```python
from build123d import *

# Parameters (mm, degrees)
SKETCH1_W           = 50
SKETCH1_H           = 10
SKETCH1_R           = 2.25
BOSS_EXTRUDE1_DEPTH = 5
SKETCH3_R           = 2.3
BOSS_EXTRUDE2_DEPTH = 10


with BuildPart() as part:
    # Sketch1 → Boss-Extrude1 (new body)
    with BuildSketch(Plane(origin=(0, 0, 0), x_dir=(1, 0, 0), z_dir=(0, 1, 0))):
        Rectangle(SKETCH1_W, SKETCH1_H)
        with Locations((-20, 0)):
            Circle(SKETCH1_R, mode=Mode.SUBTRACT)
        with Locations((20, 0)):
            Circle(SKETCH1_R, mode=Mode.SUBTRACT)
    extrude(amount=BOSS_EXTRUDE1_DEPTH)

    # Sketch3 → Boss-Extrude2 (add)
    with BuildSketch(Plane.XY.offset(5)):
        with BuildLine():
            Line((-5, 5), (-5, 9))
            ThreePointArc((-5, 9), (0, 14), (5, 9))
            Line((5, 9), (5, 5))
            Line((5, 5), (-5, 5))
        make_face()
        with Locations((0, 9)):
            Circle(SKETCH3_R, mode=Mode.SUBTRACT)
    extrude(amount=-BOSS_EXTRUDE2_DEPTH)


solid = part.part
```
CAD build for the part. Positions are in the model's coordinates, mm. A direction names the side the tool comes from. Coordinates: 2 decimals unless noted, no trailing zeros. Order: outer loops, then holes, each group sorted by start corner. A loop starts at its lowest first (then second) coordinate and runs counter-clockwise, first axis right, second up. Notation, with made-up numbers: M -29,45.25 L -3,45.25 A21 ccw -3,56.25 Z; hole C 30.5,73 d8. An arc over 180 degrees is marked long. Write each question's results on one line, items separated by ' | '. Start each with the question number.
Q1. Which spindle directions (+Z, -Z, +X, -X, +Y, -Y) get a long thin tool onto all of the face, cutting with end or side? Do faces 1 (the flat face through (-15, 5, 0)), 2 (the cylindrical face through (-17.854, 2.465, -0.676)), 3 (the flat face through (5, 7, 0)). Say none if no direction does.
Q2. Flat gauge pins, fed straight in: P1, Ø2, axis at y = 6.5, z = 0, coming from the -X side; P2, Ø2, axis at x = -6.5, z = 1, coming from the +Y side; P3, Ø2, axis at y = 12.5, z = 0.5, coming from the -X side. Where does each tip first touch, or does it go through?
Q3. Cut at B-B (x = 0). List the corners of the cut face in (y, z), then the cut area to 3 significant figures.
Q4. Cut at A-A (z = 0). List the corners of the cut face in (x, y), then the cut area to 3 significant figures.
Q5. Cut at C-C (y = 4). List the corners of the cut face in (x, z).
Q6. Cut at D-D (z = 3.5). List the corners of the cut face in (x, y), then the cut area to 3 significant figures.
Q7. Drill centre lines: probe 1 along X at (y, z) = (3.2, 0); probe 2 along Z at (x, y) = (-20, 1.7); probe 3 along Y at (x, z) = (0, -0.5). Where is each one in solid material? Low to high. Write a range as from..to.
Q8. Pull direction Z, two halves, no side cores. Call faces 4 (the flat face through (0, 2, -5)), 5 (the cylindrical face through (22.146, 2.465, -0.676)), 6 (the flat face through (25, 2, 0)): +Z half, -Z half, draft (parallel to the pull), parting line (faces both ways), or undercut.
Found:
1) face 1: +Z, -Z, -X, +Y | face 2: +Y, -Y | face 3: +Z, -Z, +X, +Y
2) P1: x = -5 | P2: y = 5 | P3: x = -4.33
3) outline: M 0,-5 L 6.7,-5 L 6.7,5 L 0,5 Z; M 11.3,-5 L 14,-5 L 14,5 L 11.3,5 Z | area: 94.0 mm²
4) outline: M -25,0 L -22.25,0 L -22.25,5 L -25,5 Z; M -17.75,0 L 17.75,0 L 17.75,5 L 5,5 L 5,9 A5 ccw -5,9 L -5,5 L -17.75,5 Z; M 22.25,0 L 25,0 L 25,5 L 22.25,5 Z; hole C 0,9 d4.6 | area: 268 mm²
5) outline: M -25,-5 L 25,-5 L 25,5 L -25,5 Z; hole C -20,0 d4.5; hole C 20,0 d4.5
6) outline: M -25,0 L 25,0 L 25,5 L 5,5 L 5,9 A5 ccw -5,9 L -5,5 L -25,5 Z; hole C 0,9 d4.6 | area: 313 mm²
7) probe 1: -25..-22.25, -17.75..17.75, 22.25..25 | probe 2: -5..-2.25, 2.25..5 | probe 3: 0..6.7, 11.3..14
8) face 4: -Z half | face 5: undercut | face 6: draft
